```python
from build123d import *
from build123d.topology import SkipClean

# Parameters (mm, degrees)
SKETCH_1_W      = 52
SKETCH_1_H      = 52
EXTRUDE_1_DEPTH = 3


with BuildPart() as part:
    # 草图1 → 凸台-拉伸1 (new body)
    with BuildSketch(Plane(origin=(0, 0, 0), x_dir=(1, 0, 0), z_dir=(0, 1, 0))):
        with BuildLine():
            Line((-140, -50), (-70, -50))
            Line((-70, -50), (-70, 25))
            Line((-70, 25), (0, 25))
            Line((0, 25), (0, 33.5))
            ThreePointArc((0, 33.5), (-1.5, 35), (0, 36.5))
            Line((0, 36.5), (0, 67))
            ThreePointArc((0, 67), (-3, 70), (0, 73))
            Line((0, 73), (0, 78.5))
            ThreePointArc((0, 78.5), (-1.5, 80), (0, 81.5))
            Line((0, 81.5), (0, 95))
            Line((0, 95), (-98.740841322, 95))
            Line((-98.740841322, 95), (-118.732050781, 115.024358473))
            Line((-118.732050781, 115.024358473), (-164.024358473, 69.80702923))
            Line((-164.024358473, 69.80702923), (-140, 45.742834058))
            Line((-140, 45.742834058), (-140, -50))
        make_face()
        Polygon((-82, 69.73908001), (-118.8, 33), (-155.53908001, 69.8), (-118.73908001, 106.53908001), align=None, mode=Mode.SUBTRACT)
        with Locations((-36, 59)):
            Rectangle(SKETCH_1_W, SKETCH_1_H, mode=Mode.SUBTRACT)
        with Locations((-108, -13)):
            Rectangle(SKETCH_1_W, SKETCH_1_H, mode=Mode.SUBTRACT)
    extrude_1 = extrude(amount=EXTRUDE_1_DEPTH)

    # 镜向1: 凸台-拉伸1 across plane
    with SkipClean():  # the faces are left unmerged after this step: merging them gives an invalid solid
        add(extrude_1.mirror(Plane(origin=(0, 3, -36.5), x_dir=(0, 0, 1), z_dir=(-1, 0, 0))))


solid = part.part
```
Could you check a few things on this model? Use its own coordinates, in mm. A direction names the side the tool comes from. Coordinates: 2 decimals unless noted, no trailing zeros. Order: outer loops, then holes, each group sorted by start corner. A loop starts at its lowest first (then second) coordinate and runs counter-clockwise, first axis right, second up. Notation, with made-up numbers: M 44,89.25 L 101,89.25 A28 ccw 101,128.25 Z; hole C 67,81 d1. An arc over 180 degrees is marked long. Use one line per item in the form item = value. Start each with the question number.
1. We'd pull the mould along X, two halves only. Please class faces 4 (the flat face through (-100.14, 1.48, -51.63)), 5 (the flat face through (-141.061, 1.479, -92.732)), 6 (the flat face through (-100.63, 1.48, -88.4)), 7 (the flat face through (2, 0, -34)): +X half, -X half, draft (parallel to the pull), parting line (faces both ways), or undercut.
2. Suppose I cut it at D-D on x = -105. Write out the boundary of the cut face in (y, z).
3. For pin 1 (1.5 mm diameter, centred on y = 1, z = 26, fed in from -X); pin 2 (0.9 mm diameter, centred on y = 1, z = 11, fed in from +X); pin 3 (1 mm diameter, centred on x = 5.5, y = 1.5, fed in from +Z), each with a flat end and sliding along its axis, tell me the tip position at first contact or that it passes through.
4. On a 3-axis mill with a long thin cutter (end or side, diameter ignored), from which of +Z, -Z, +X, -X, +Y, -Y can I reach the whole of each face in a straight line? I mean faces 1 (the flat face through (108.597, 1.479, -104.872)), 2 (the flat face through (-137.4, 1.48, -87.91)), 3 (the flat face through (-152.18, 1.479, -57.943)). Say none if no direction works.
5. Suppose I cut it at C-C on z = 0.5. Write out the boundary of the cut face in (x, y), then the cut area to 3 significant figures.
6. Suppose I cut it at A-A on x = -19. Write out the boundary of the cut face in (y, z), then the cut area to 3 significant figures.
7. Suppose I cut it at B-B on z = -22. Write out the boundary of the cut face in (x, y).
8. Please list where these lines run through material, in increasing order: line 1 (Z direction, x = 0, y = 1.75); line 2 (X direction, y = 2.6, z = 32.5); line 3 (X direction, y = 1.5, z = -70).
Geometry says:
q1.face_4 = undercut
q1.face_5 = -X half
q1.face_6 = undercut
q1.face_7 = draft
q2.outline = M 0,-101.27 L 3,-101.27 L 3,-92.78 L 0,-92.78 Z; M 0,-46.78 L 3,-46.78 L 3,-13 L 0,-13 Z; M 0,39 L 3,39 L 3,50 L 0,50 Z
q3.pin_1 = -140
q3.pin_2 = 140
q3.pin_3 = -25
q4.face_1 = -Z, +Y, -Y
q4.face_2 = +Y, -Y
q4.face_3 = +Z, -X, +Y, -Y
q5.outline = M -140,0 L -134,0 L -134,3 L -140,3 Z; M -82,0 L -70,0 L -70,3 L -82,3 Z; M 70,0 L 82,0 L 82,3 L 70,3 Z; M 134,0 L 140,0 L 140,3 L 134,3 Z
q5.area = 108 mm^2
q6.outline = M 0,-95 L 3,-95 L 3,-85 L 0,-85 Z; M 0,-33 L 3,-33 L 3,-25 L 0,-25 Z
q6.area = 54.0 mm^2
q7.outline = M -140,0 L -70,0 L -70,3 L -140,3 Z; M 70,0 L 140,0 L 140,3 L 70,3 Z
q8.line_1 = -95 to -81.5, -78.5 to -73, -67 to -36.5, -33.5 to -25
q8.line_2 = -140 to -134, -82 to -70, 70 to 82, 134 to 140
q8.line_3 = -163.83 to -155.34, -82.26 to -62, -10 to -3, 3 to 10, 62 to 82.26, 155.34 to 163.83
